Geometry: final body of the model. Coordinates: model frame, mm. Face numbers are marked on the shaded views. A direction names the side the tool comes from. Round coordinates to 2 decimals unless told otherwise and drop trailing zeros. Write each loop counter-clockwise with the first axis right and the second up, starting at its lowest first coordinate (ties: lowest second). Pieces come first, ordered by that corner, then holes. Notation, with made-up numbers: M -14.5,48.5 L 25.5,48.5 A20 cw 25.5,72.5 Z; hole C 61,31 d2. An arc over 180 degrees is marked long. Put each result on its own line as item: value. Start each with the question number.
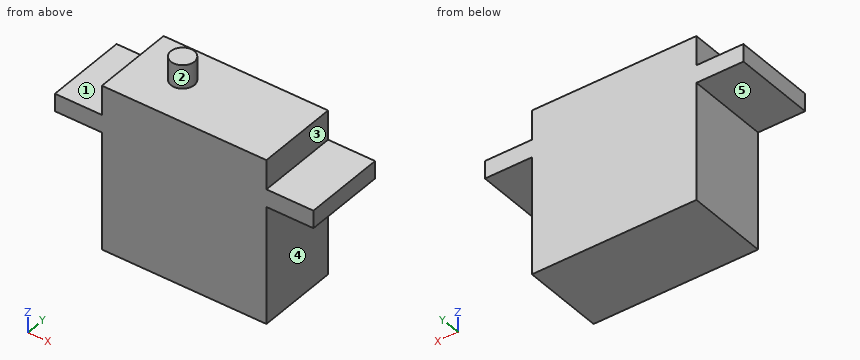
```python
from build123d import *

# Parameters (mm, degrees)
F0_W     = 22.225
F0_H     = 22.225
F1_DEPTH = 11.1125
F2_W     = 11.1125
F2_H     = 2.38125
F3_DEPTH = 6.35
F4_W     = 11.1125
F4_H     = 2.38125
F5_DEPTH = 6.35
F6_R     = 1.5875
F7_DEPTH = 3.175


with BuildPart() as f1:
    # F0 (on Front) → F1 (new body)
    with BuildSketch(Plane.XZ):
        with Locations((11.1125, -11.1125)):
            Rectangle(F0_W, F0_H)
    extrude(amount=F1_DEPTH)

    # F2 (on face) → F3 (join)
    with BuildSketch(Plane.YZ.offset(22.225)):
        with Locations((-5.55625, -5.159375)):
            Rectangle(F2_W, F2_H)
    extrude(amount=F3_DEPTH)

    # F4 (on face) → F5 (join)
    with BuildSketch(Plane(origin=(0, 0, 0), x_dir=(0, -1, 0), z_dir=(-1, 0, 0))):
        with Locations((5.55625, -5.159375)):
            Rectangle(F4_W, F4_H)
    extrude(amount=F5_DEPTH)

    # F6 (on face) → F7 (join)
    with BuildSketch(Plane.XY):
        with Locations((6.35, -5.039688)):
            Circle(F6_R)
    extrude(amount=F7_DEPTH)


solid = f1.part
```
1) Section B-B, the plane x = 6.35. Output: boundary loops of the cut face in (y, z) (1 decimal), and give its area (3 significant figures).
2) Access query for the marked faces 1, 2, 3, 4 and 5. Directions: +Z, -Z, +X, -X, +Y, -Y. A direction counts if a zero-diameter tool reaches every point of the face in a straight line with its end or side. Return the directions, or none.
3) Ray query, probe 1 along Z at (x, y) = (13, -2) (3 decimals); probe 2 along X at (y, z) = (-6, -12.5) (3 decimals); probe 3 along Z at (x, y) = (23, -2.25). Return the intervals inside material, ascending.
4) First-contact query: pin 1 (6 mm diameter, centred on x = 11, z = -7, fed in from +Y); pin 2 (1.5 mm diameter, centred on x = 18.5, y = -6.5, fed in from +Z); pin 3 (1.9 mm diameter, centred on x = 26, y = -5, fed in from +Z); pin 4 (3.5 mm diameter, centred on y = -3.5, z = -11, fed in from -X). Flat tips, straight axial feed; report the tip coordinate or a pass-through.
5) Section D-D, the plane x = -2.5. Output: boundary loops of the cut face in (y, z).
6) Section A-A, the plane y = -9.5. Output: boundary loops of the cut face in (x, z) (3 decimals).
7) Section C-C, the plane z = -9.75. Output: boundary loops of the cut face in (x, y) (1 decimal).
Solved:
1. outline: M -11.1,-22.2 L 0,-22.2 L 0,0 L -3.5,0 L -3.5,3.2 L -6.6,3.2 L -6.6,0 L -11.1,0 Z
1. area: 257 mm2
2. face 1: +Z, -X, +Y, -Y
2. face 2: +Z
2. face 3: +Z, +X, +Y, -Y
2. face 4: -Z, +X, +Y, -Y
2. face 5: -Z, -X, +Y, -Y
3. probe 1: z = -22.225 to 0
3. probe 2: x = 0 to 22.225
3. probe 3: z = -6.35 to -3.97
4. pin 1: stops at y = 0
4. pin 2: stops at z = 0
4. pin 3: stops at z = -3.97
4. pin 4: stops at x = 0
5. outline: M -11.11,-6.35 L 0,-6.35 L 0,-3.97 L -11.11,-3.97 Z
6. outline: M -6.35,-6.35 L 0,-6.35 L 0,-22.225 L 22.225,-22.225 L 22.225,-6.35 L 28.575,-6.35 L 28.575,-3.969 L 22.225,-3.969 L 22.225,0 L 0,0 L 0,-3.969 L -6.35,-3.969 Z
7. outline: M 0,-11.1 L 22.2,-11.1 L 22.2,0 L 0,0 Z
